```python
from build123d import *

# Parameters (mm, degrees)
F0_W     = 76.2
F0_H     = 76.2
F1_DEPTH = 76.2
F3_D     = 25.4
F4_W     = 25.4
F4_H     = 25.4
F5_DEPTH = 12.7


# Not quite as in the source:
# - the program builds the solid bodies; features that only make, move or delete a surface that nothing else refers to are left out


with BuildPart() as f1:
    # F0 (on Front) → F1 (new body)
    with BuildSketch(Plane.XZ):
        with Locations((38.1, 38.1)):
            Rectangle(F0_W, F0_H)
    extrude(amount=F1_DEPTH)

    # F3 (through all)
    with Locations(Plane.XY.offset(76.2)):
        with Locations((37.7037897706, -36.2189039588)):
            Hole(F3_D / 2)

    # F4 (on face) → F5 (join)
    with BuildSketch(Plane.XZ.offset(76.2)):
        with Locations((37.6457564205, 37.7473003834)):
            Rectangle(F4_W, F4_H)
    extrude(amount=F5_DEPTH)


solid = f1.part
```
Geometry check sheet. Reference: the model listing, model coordinates, mm. A direction names the side the tool comes from. Round coordinates to 2 decimals unless told otherwise and drop trailing zeros. Write each loop counter-clockwise with the first axis right and the second up, starting at its lowest first coordinate (ties: lowest second). Pieces come first, ordered by that corner, then holes. Notation, with made-up numbers: (-19, 14.5) -> (5, 14.5) arc R27 cw to (5, 48.5) -> close; hole circle Ø3 at (39, 84). An arc over 180 degrees is marked (long way). Put each result on its own line as item: value.
1) Depth check by flat-ended pin: P1, Ø10, axis at x = 37, y = -83, coming from the +Z side; P2, Ø15, axis at x = 37.7, y = -36.22, coming from the -Z side; P3, Ø6.5, axis at y = -80, z = 39.5, coming from the +X side; P4, Ø6, axis at x = 26.5, z = 14.5, coming from the -Y side. Enter the tip coordinate at first touch or a pass-through.
Recorded:
P1: stops at z = 50.45
P2: passes through
P3: stops at x = 50.35
P4: stops at y = -76.2
2) Cross-section at D-D, the plane x = 13. Enter the section's corners in (y, z), plus the area to 3 significant figures.
Recorded:
outline: (-76.2, 0) -> (0, 0) -> (0, 76.2) -> (-76.2, 76.2) -> close
area: 5,810 mm2
3) Cross-section at C-C, the plane y = -82. Enter the section's corners in (x, z), plus the area to 3 significant figures.
Recorded:
outline: (24.95, 25.05) -> (50.35, 25.05) -> (50.35, 50.45) -> (24.95, 50.45) -> close
area: 645 mm2
4) Cross-section at B-B, the plane z = 26.5. Enter the section's corners in (x, y), plus the area to 3 significant figures.
Recorded:
outline: (0, -76.2) -> (24.95, -76.2) -> (24.95, -88.9) -> (50.35, -88.9) -> (50.35, -76.2) -> (76.2, -76.2) -> (76.2, 0) -> (0, 0) -> close; hole circle Ø25.4 at (37.7, -36.22)
area: 5,620 mm2
5) Thickness scan on probe 1 along Z at (x, y) = (43, -83.5); probe 2 along Y at (x, z) = (70, 24); probe 3 along Y at (x, z) = (28, 20). Record the ranges inside material, lowest first. Write a range as from..to.
Recorded:
probe 1: z = 25.05..50.45
probe 2: y = -76.2..0
probe 3: y = -76.2..-44.41, -28.03..0
6) Cross-section at A-A, the plane x = 46.5. Enter the section's corners in (y, z).
Recorded:
outline: (-88.9, 25.05) -> (-76.2, 25.05) -> (-76.2, 0) -> (-45.38, 0) -> (-45.38, 76.2) -> (-76.2, 76.2) -> (-76.2, 50.45) -> (-88.9, 50.45) -> close; (-27.06, 0) -> (0, 0) -> (0, 76.2) -> (-27.06, 76.2) -> close
7) Access from +Z, -Z, +X, -X, +Y, -Y to the whole of each face (thin tool, end or side, straight path). Record for faces 4 (the face through (24.946, -82, 38)), 5 (the face through (37, -82, 50.447)), 6 (the face through (37, -88.9, 38)).
Recorded:
face 4: +Z, -Z, -X, -Y
face 5: +Z, +X, -X, -Y
face 6: +Z, -Z, +X, -X, -Y
8) Release check for a two-part mould opening along X. For faces 1 (the face through (50.346, -82, 38)), 2 (the face through (37, -82, 25.047)), 3 (the face through (31.844, -47.486, 37.567)) record: pulls with the +X half, pulls with the -X half, needs draft (parallel to the pull), parting line crosses it, or undercut.
Recorded:
face 1: pulls with the +X half
face 2: needs draft
face 3: undercut
